from build123d import *

# Parameters (mm, degrees)
SKETCH2_W           = 63.5
SKETCH2_H           = 63.5
BOSS_EXTRUDE1_DEPTH = 241.3
SKETCH4_W           = 50.8
SKETCH4_H           = 50.8
CUT_EXTRUDE1_DEPTH  = 95.25
SKETCH5_R           = 6.35
CUT_EXTRUDE2_DEPTH  = 64.5
SKETCH6_R           = 6.35
CUT_EXTRUDE3_DEPTH  = 12.7
CUT_EXTRUDE4_DEPTH  = 7.35
CUT_EXTRUDE6_START  = -31.75
CUT_EXTRUDE6_DEPTH  = 31.75
SKETCH37_W          = 8.89
SKETCH37_H          = 10.16
BOSS_EXTRUDE3_DEPTH = 10.16
SKETCH38_R          = 2.032
CUT_EXTRUDE8_DEPTH  = 58.674
FILLET4_R           = 3.81
SKETCH40_R          = 11.176
CUT_EXTRUDE10_DEPTH = 12.7


with BuildPart() as part:
    # Sketch2 → Boss-Extrude1 (new body)
    with BuildSketch(Plane(origin=(0, 0, 0), x_dir=(1, 0, 0), z_dir=(0, 1, 0))):
        with Locations((-9.601422319, 6.627899344)):
            Rectangle(SKETCH2_W, SKETCH2_H)
    extrude(amount=BOSS_EXTRUDE1_DEPTH)

    # Sketch4 → Cut-Extrude1 (cut, symmetric)
    with BuildSketch(Plane(origin=(0, 101.6, 0), x_dir=(1, 0, 0), z_dir=(0, 1, 0))):
        with Locations((-15.951422319, 12.977899344)):
            Rectangle(SKETCH4_W, SKETCH4_H)
    extrude(amount=CUT_EXTRUDE1_DEPTH, both=True, mode=Mode.SUBTRACT)

    # Sketch5 → Cut-Extrude2 (cut, through all)
    with BuildSketch(Plane.XY.offset(25.122100656)):
        with Locations((-15.951422319, 25.4)):
            Circle(SKETCH5_R)
        with Locations((-15.951422319, 50.8)):
            Circle(SKETCH5_R)
        with Locations((-15.951422319, 76.2)):
            Circle(SKETCH5_R)
        with Locations((-15.951422319, 101.6)):
            Circle(SKETCH5_R)
        with Locations((-15.951422319, 127)):
            Circle(SKETCH5_R)
        with Locations((-15.951422319, 152.4)):
            Circle(SKETCH5_R)
        with Locations((-15.951422319, 177.8)):
            Circle(SKETCH5_R)
    extrude(amount=-CUT_EXTRUDE2_DEPTH, mode=Mode.SUBTRACT)

    # Sketch6 → Cut-Extrude3 (cut)
    with BuildSketch(Plane(origin=(22.148577681, 0, 0), x_dir=(0, 0, -1), z_dir=(1, 0, 0))):
        with Locations((2.817899344, 12.7)):
            Circle(SKETCH6_R)
        with Locations((2.817899344, 38.1)):
            Circle(SKETCH6_R)
        with Locations((2.817899344, 63.5)):
            Circle(SKETCH6_R)
        with Locations((2.817899344, 88.9)):
            Circle(SKETCH6_R)
        with Locations((2.817899344, 114.3)):
            Circle(SKETCH6_R)
        with Locations((2.817899344, 139.7)):
            Circle(SKETCH6_R)
        with Locations((2.817899344, 165.1)):
            Circle(SKETCH6_R)
        with Locations((2.817899344, 190.5)):
            Circle(SKETCH6_R)
    extrude(amount=-CUT_EXTRUDE3_DEPTH, mode=Mode.SUBTRACT)

    # Sketch7 → Cut-Extrude4 (cut, through all)
    with BuildSketch(Plane(origin=(0, 6.35, 0), x_dir=(1, 0, 0), z_dir=(0, 1, 0))):
        Polygon((-41.351422319, 38.377899344), (9.448577681, 38.377899344), (9.448577681, 0.277899344), (9.448577681, -12.422100656), (-3.251422319, -12.422100656), (-41.351422319, -12.422100656), align=None)
    extrude(amount=-CUT_EXTRUDE4_DEPTH, mode=Mode.SUBTRACT)

    # Sketch34 → Cut-Extrude6 (cut)
    with BuildSketch(Plane.XZ.offset(-196.85).offset(CUT_EXTRUDE6_START)):
        Polygon((-3.251422319, 12.422100656), (9.448577681, 12.422100656), (9.448577681, -0.277899344), (9.448577681, -38.377899344), (-41.351422319, -38.377899344), (-41.351422319, 12.422100656), align=None)
    extrude(amount=CUT_EXTRUDE6_DEPTH, mode=Mode.SUBTRACT)

    # Sketch37 → Boss-Extrude3 (add)
    with BuildSketch(Plane(origin=(0, 228.6, 0), x_dir=(1, 0, 0), z_dir=(0, 1, 0))):
        with Locations((-32.080422319, 2.817899344)):
            Rectangle(SKETCH37_W, SKETCH37_H)
        with Locations((-15.316422319, 2.817899344)):
            Rectangle(SKETCH37_W, SKETCH37_H)
    extrude(amount=-BOSS_EXTRUDE3_DEPTH)

    # Sketch38 → Cut-Extrude8 (cut)
    with BuildSketch(Plane.ZY.offset(36.525422319)):
        with Locations((-2.817899344, 223.52)):
            Circle(SKETCH38_R)
    extrude(amount=-CUT_EXTRUDE8_DEPTH, mode=Mode.SUBTRACT)

    # Fillet4
    fillet4_edges = [part.edges().sort_by_distance(p)[0] for p in [
        (-32.080422319, 218.44, -7.897899344),
        (-32.080422319, 218.44, 2.262100656),
        (-15.316422319, 218.44, -7.897899344),
        (-15.316422319, 218.44, 2.262100656),
    ]]
    fillet(fillet4_edges, radius=FILLET4_R)

    # Sketch40 → Cut-Extrude10 (cut)
    with BuildSketch(Plane(origin=(22.148577681, 0, 0), x_dir=(0, 0, -1), z_dir=(1, 0, 0))):
        with Locations((0.277899344, 215.9)):
            Circle(SKETCH40_R)
    extrude(amount=-CUT_EXTRUDE10_DEPTH, mode=Mode.SUBTRACT)


solid = part.part
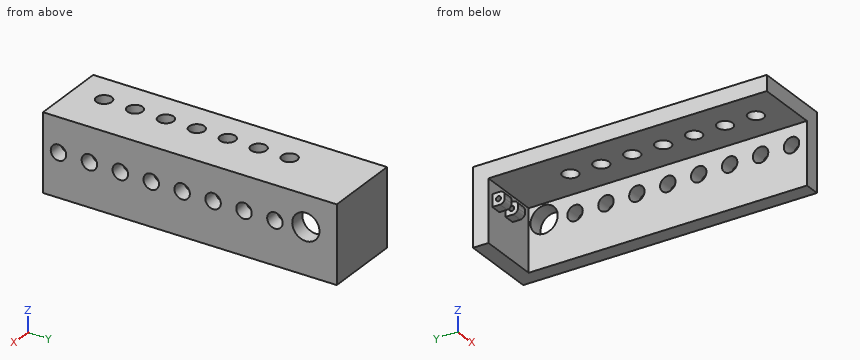
Design review of the part built by this model. Coordinates are the model's own, in mm. Give positions to 0.01 mm unless a question says otherwise; leave off trailing zeros. Loops run counter-clockwise (first coordinate to the right, second up) from the corner with the lowest first, then second, coordinate; pieces in that order, holes last. Notation, with made-up numbers: M 6.5,-2.75 L 31.5,-2.75 A28 ccw 31.5,19.25 Z; hole C -32.5,-38 d2. An arc over 180 degrees is marked long. One line per question, with ' | ' between items. Start each with the question number.
1. Add section B-B (z = 18). Write out the cut boundary in (x, y), plus the area to 3 significant figures.
2. To check wall thickness, follow L1, parallel to Z at x = -15.25, y = 223.52; L2, parallel to X at y = 101, z = 19; L3, parallel to Z at x = 17, y = 12. State the ranges of each line that lie inside material, in increasing order.
3. Insertion check: P1, Ø1, axis at x = -22, y = 126, coming from the -Z side; P2, Ø1.9, axis at x = -33, y = 227, coming from the -Z side; P3, Ø8, axis at y = 223, z = -3.5, coming from the -X side. Each pin has a flat end and moves straight along its axis. Give the tip position at first contact, or say it passes through.
4. Add section D-D (x = -4). Write out the cut boundary in (y, z).
5. Add section A-A (y = 101.6). Write out the cut boundary in (x, z), plus the area to 3 significant figures.
6. Add section C-C (z = 8). Write out the cut boundary in (x, y).
Worked out:
1) outline: M -41.35,0 L 22.15,0 L 22.15,241.3 L -41.35,241.3 Z; hole C -15.95,25.4 d12.7; hole C -15.95,50.8 d12.7; hole C -15.95,76.2 d12.7; hole C -15.95,101.6 d12.7; hole C -15.95,127 d12.7; hole C -15.95,152.4 d12.7; hole C -15.95,177.8 d12.7 | area: 14,400 mm²
2) L1: z = -7.9 to -4.85, -0.79 to 2.26, 12.42 to 25.12 | L2: x = -41.35 to -22.27, -9.63 to 22.15 | L3: z = -38.38 to -9.13, 3.49 to 25.12
3) P1: stops at z = 12.42 | P2: stops at z = -7.9 | P3: stops at x = -36.53
4) outline: M 0,12.42 L 228.6,12.42 L 228.6,-38.38 L 241.3,-38.38 L 241.3,25.12 L 0,25.12 Z
5) outline: M -41.35,12.42 L -22.3,12.42 L -22.3,25.12 L -41.35,25.12 Z; M -9.6,12.42 L 9.45,12.42 L 9.45,-38.38 L 22.15,-38.38 L 22.15,25.12 L -9.6,25.12 Z | area: 1,290 mm²
6) outline: M -41.35,228.6 L 9.45,228.6 L 9.45,223.41 L 22.15,223.41 L 22.15,241.3 L -41.35,241.3 Z; M 9.45,0 L 22.15,0 L 22.15,208.39 L 9.45,208.39 Z
